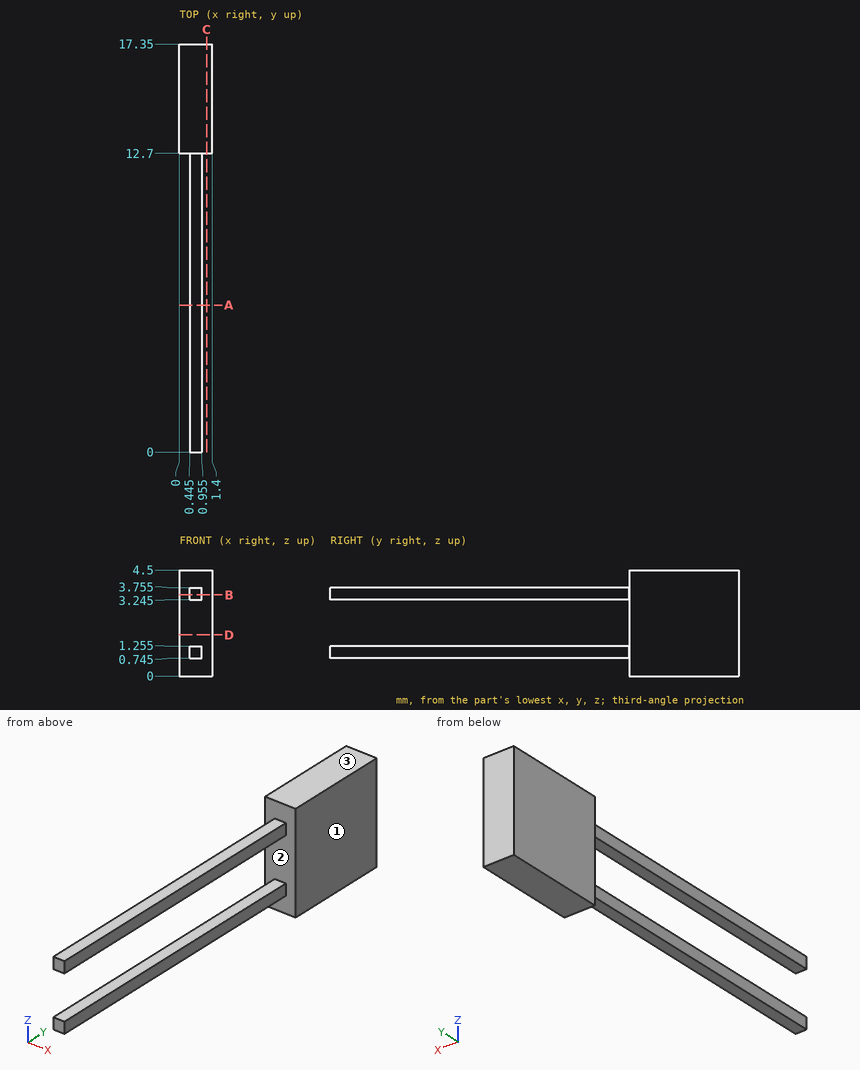
Design review of the part shown in the three views and the two pictorial views. Dimensions are in mm from the part's minimum x, y and z. Give positions to 0.01 mm unless a question says otherwise; leave off trailing zeros. Loops run counter-clockwise (first coordinate to the right, second up) from the corner with the lowest first, then second, coordinate; pieces in that order, holes last. Notation, with made-up numbers: M 26,41 L 64,41 A14 ccw 64,58 Z; hole C -32.5,-13.5 d10. An arc over 180 degrees is marked long. Put each result on its own line as item: value. Start each with the question number.
(1) Add section B-B, the plane z = 3.45. Write out the cut boundary in (x, y) (3 decimals).
(2) Add section A-A, the plane y = 6.25. Write out the cut boundary in (x, z) (3 decimals), then the cut area to 3 significant figures.
(3) For pin 1 (0.6 mm diameter, centred on x = 1, y = 9.5, fed in from -Z) (3 decimals); pin 2 (0.7 mm diameter, centred on x = 1, z = 3, fed in from -Y); pin 3 (1 mm diameter, centred on y = 2.5, z = 3.5, fed in from +X) (3 decimals), all flat-tipped, find the tip position at first contact; note any pin that passes through.
(4) The part is to be moulded in two halves that separate along Z. For the marked faces 1, 2 and 3, say which applies: +Z half, -Z half, draft (parallel to the pull), parting line (faces both ways), or undercut.
(5) Add section C-C, the plane x = 1.15. Write out the cut boundary in (y, z), then the cut area to 3 significant figures.
(6) Wall thickness on L1, parallel to Z at x = 0.5, y = 5 (3 decimals); L2, parallel to Y at x = 0.15, z = 4.1; L3, parallel to X at y = 10.75, z = 3.6 (3 decimals): over which ranges is each line inside the solid? List them lowest first.
(7) Add section D-D, the plane z = 1.75. Write out the cut boundary in (x, y), then the cut area to 3 significant figures.
Result:
1. outline: M 0,12.7 L 0.445,12.7 L 0.445,0 L 0.955,0 L 0.955,12.7 L 1.4,12.7 L 1.4,17.35 L 0,17.35 Z
2. outline: M 0.445,0.745 L 0.955,0.745 L 0.955,1.255 L 0.445,1.255 Z; M 0.445,3.245 L 0.955,3.245 L 0.955,3.755 L 0.445,3.755 Z
2. area: 0.520 mm^2
3. pin 1: stops at z = 0.745
3. pin 2: stops at y = 0
3. pin 3: stops at x = 0.955
4. face 1: draft
4. face 2: undercut
4. face 3: +Z half
5. outline: M 12.7,0 L 17.35,0 L 17.35,4.5 L 12.7,4.5 Z
5. area: 20.9 mm^2
6. L1: z = 0.745 to 1.255, 3.245 to 3.755
6. L2: y = 12.7 to 17.35
6. L3: x = 0.445 to 0.955
7. outline: M 0,12.7 L 1.4,12.7 L 1.4,17.35 L 0,17.35 Z
7. area: 6.51 mm^2
